Here's how the part is built. I have some questions about the finished solid (model axes, mm). Face numbers are marked on the shaded views. A direction names the side the tool comes from. Coordinates: 2 decimals unless noted, no trailing zeros. Order: outer loops, then holes, each group sorted by start corner. A loop starts at its lowest first (then second) coordinate and runs counter-clockwise, first axis right, second up. Notation, with made-up numbers: (61.5, 37.25) - (104.5, 37.25) arc R25 cw to (104.5, 72.25) - close; hole circle Ø1 at (21.5, -31.5). An arc over 180 degrees is marked (long way). Answer as CSV lines item,"result". Start each with the question number.
Q1. Suppose I cut it at B-B (x = -3.5). Please give me the cut outline in (y, z), then the cut area to 3 significant figures.
Q2. For pin 1 Ø11.5 at (x, y) = (-7.5, -6) entering from +Z, with a flat end and sliding along its axis, tell me the tip position at first contact or that it passes through.
Q3. Suppose I cut it at C-C (y = -1). Please give me the cut outline in (x, z), then the cut area to 3 significant figures.
Q4. Thinking about a two-plate mould opening in X: for the marked faces 3, 4, 5 and 6, which applies, released by +X, released by -X, zero draft, split by the parting line, or undercut?
Q5. Suppose I cut it at A-A (z = 5.2). Please give me the cut outline in (x, y).
Q6. For the marked faces 1 and 2, which set-ups out of +Z, -Z, +X, -X, +Y, -Y let a thin tool reach every point of the face, with its end or its side?
Q7. I need wall thicknesses on line 1 (X direction, y = -10.5, z = 5.5); line 2 (X direction, y = 2.5, z = 4.3); line 3 (Y direction, x = -11.5, z = 1.85). Which ranges of each line are inside material? Lowest first, please.
Q8. Suppose I cut it at D-D (y = -11.5). Please give me the cut outline in (x, z).
from build123d import *

# Parameters (mm, degrees)
F0_W     = 22.6
F0_H     = 22.6
F0_R     = 1.25
F1_DEPTH = 1.2
F0_W_2   = 25
F0_H_2   = 25
F2_DEPTH = 6


with BuildPart() as f1:
    # F0 (on Top) → F1 (new body)
    with BuildSketch(Plane.XY):
        with Locations((-8.805462, -6.924062)):
            Rectangle(F0_W, F0_H)
        with Locations((-1.105462, -10.624062)):
            Circle(F0_R, mode=Mode.SUBTRACT)
        with Locations((-16.105462, -3.224062)):
            Circle(F0_R, mode=Mode.SUBTRACT)
    extrude(amount=F1_DEPTH)

    # F0 (on Top) → F2 (join)
    with BuildSketch(Plane.XY):
        with Locations((-8.805462, -6.924062)):
            Rectangle(F0_W_2, F0_H_2)
        with Locations((-8.805462, -6.924062)):
            Rectangle(F0_W, F0_H, mode=Mode.SUBTRACT)
        with Locations((-16.105462, -3.224062)):
            Circle(F0_R)
        with Locations((-1.105462, -10.624062)):
            Circle(F0_R)
    extrude(amount=F2_DEPTH)


solid = f1.part
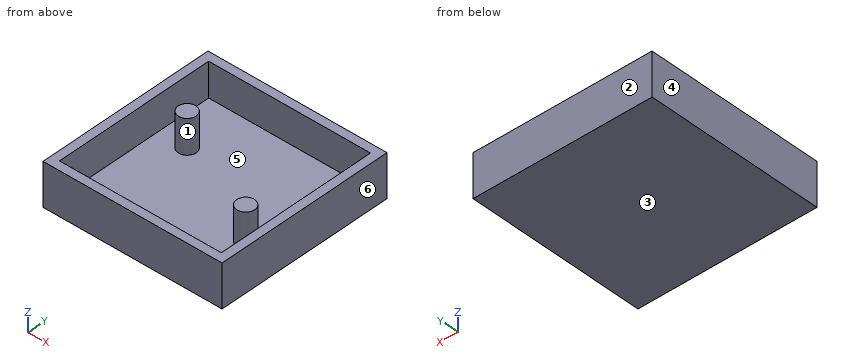
Here are the results:
1,outline,"(-19.42, 0) - (5.58, 0) - (5.58, 6) - (4.38, 6) - (4.38, 1.2) - (-18.22, 1.2) - (-18.22, 6) - (-19.42, 6) - close"
1,area,"41.5 mm²"
2,pin 1,"stops at z = 1.2"
3,outline,"(-21.31, 0) - (3.69, 0) - (3.69, 6) - (2.49, 6) - (2.49, 1.2) - (-20.11, 1.2) - (-20.11, 6) - (-21.31, 6) - close"
3,area,"41.5 mm²"
4,face 3,"zero draft"
4,face 4,"released by -X"
4,face 5,"undercut"
4,face 6,"released by +X"
5,outline,"(-21.31, -19.42) - (3.69, -19.42) - (3.69, 5.58) - (-21.31, 5.58) - close; circle Ø2.5 at (-16.11, -3.22); circle Ø2.5 at (-1.11, -10.62); hole (-20.11, -18.22) - (2.49, -18.22) - (2.49, 4.38) - (-20.11, 4.38) - close"
6,face 1,"+Z"
6,face 2,"+Z, -Z, +X, -X, +Y"
7,line 1,"x = -21.31 to -20.11, -2.35 to 0.14, 2.49 to 3.69"
7,line 2,"x = -21.31 to -20.11, 2.49 to 3.69"
7,line 3,"y = -19.42 to -18.22, 4.38 to 5.58"
8,outline,"(-21.31, 0) - (3.69, 0) - (3.69, 6) - (2.49, 6) - (2.49, 1.2) - (-0.21, 1.2) - (-0.21, 6) - (-2, 6) - (-2, 1.2) - (-20.11, 1.2) - (-20.11, 6) - (-21.31, 6) - close"
